Read the model definition and answer for the solid it produces. Units are mm, in the model's axes. A direction names the side the tool comes from. Give positions to 0.01 mm unless a question says otherwise; leave off trailing zeros. Loops run counter-clockwise (first coordinate to the right, second up) from the corner with the lowest first, then second, coordinate; pieces in that order, holes last. Notation, with made-up numbers: M 61.25,61.5 L 116.25,61.5 A26 cw 116.25,93.5 Z; hole C 44,-1.75 d7. An arc over 180 degrees is marked long. Return JSON: item names as keys, results as strings. Group by question number.
```python
from build123d import *

# Parameters (mm, degrees)
EXTRUDE_1_DEPTH        = 40
SKETCH_2_W             = 70
SKETCH_2_H             = 41
EXTRUDE_2_DEPTH        = 1
SKETCH_3_W             = 70
SKETCH_3_H             = 41
EXTRUDE_3_DEPTH        = 1
SKETCH_4_R             = 2.1
CUT_EXTRUDE_1_DEPTH    = 1
CUT_EXTRUDE_2_DEPTH    = 1
CUT_EXTRUDE_3_DEPTH    = 81
PATTERN_LINEAR_1_COUNT = 3
PATTERN_LINEAR_1_PITCH = 15
CUT_EXTRUDE_4_DEPTH    = 1
PATTERN_LINEAR_2_COUNT = 3
PATTERN_LINEAR_2_PITCH = 15
SKETCH_8_W             = 68
SKETCH_8_H             = 18
CUT_EXTRUDE_5_DEPTH    = 10
FILLET_1_R             = 10


with BuildPart() as part:
    # 草图1 → 凸台-拉伸1 (new body)
    with BuildSketch(Plane(origin=(0, 0, 0), x_dir=(0, 0, -1), z_dir=(1, 0, 0))):
        Polygon((0, 0), (10, 0), (10, 40), (80, 40), (80, 0), (90, 0), (90, -1), (79, -1), (79, 39), (11, 39), (11, -1), (0, -1), align=None)
    extrude(amount=EXTRUDE_1_DEPTH)

    # 草图2 → 凸台-拉伸2 (add)
    with BuildSketch(Plane(origin=(40, 0, 0), x_dir=(0, 0, -1), z_dir=(1, 0, 0))):
        with Locations((45, 19.5)):
            Rectangle(SKETCH_2_W, SKETCH_2_H)
    extrude(amount=-EXTRUDE_2_DEPTH)

    # 草图3 → 凸台-拉伸3 (add)
    with BuildSketch(Plane.ZY):
        with Locations((-45, 19.5)):
            Rectangle(SKETCH_3_W, SKETCH_3_H)
    extrude(amount=-EXTRUDE_3_DEPTH)

    # 草图4 → 切除-拉伸1 (cut)
    with BuildSketch(Plane(origin=(0, 0, 0), x_dir=(1, 0, 0), z_dir=(0, 1, 0))):
        with Locations((5, 85)):
            Circle(SKETCH_4_R)
        with Locations((35, 85)):
            Circle(SKETCH_4_R)
        with Locations((35, 5)):
            Circle(SKETCH_4_R)
        with Locations((5, 5)):
            Circle(SKETCH_4_R)
    extrude(amount=-CUT_EXTRUDE_1_DEPTH, mode=Mode.SUBTRACT)

    # 草图5 → 切除-拉伸2 (cut)
    with BuildSketch(Plane.ZY):
        with BuildLine():
            Line((-30, 15), (-30, -16.50263466))
            ThreePointArc((-30, -16.50263466), (-45, -31.50263466), (-60, -16.50263466))
            Line((-60, -16.50263466), (-60, 15))
            ThreePointArc((-60, 15), (-45, 30), (-30, 15))
        make_face()
    extrude(amount=-CUT_EXTRUDE_2_DEPTH, mode=Mode.SUBTRACT)

    # 草图6 → 切除-拉伸3 (cut, through all)
    with BuildSketch(Plane.XY.offset(-10)):
        with BuildLine():
            Line((6.5, 34), (6.5, 24))
            ThreePointArc((6.5, 24), (5, 22.5), (3.5, 24))
            Line((3.5, 24), (3.5, 34))
            ThreePointArc((3.5, 34), (5, 35.5), (6.5, 34))
        make_face()
        with BuildLine():
            Line((6.5, 16), (6.5, 6))
            ThreePointArc((6.5, 6), (5, 4.5), (3.5, 6))
            Line((3.5, 6), (3.5, 16))
            ThreePointArc((3.5, 16), (5, 17.5), (6.5, 16))
        make_face()
    cut_extrude_3 = extrude(amount=-CUT_EXTRUDE_3_DEPTH, mode=Mode.SUBTRACT)

    # 阵列(线性)1: 切除-拉伸3 ×3
    with Locations(*[(i * PATTERN_LINEAR_1_PITCH, 0, 0) for i in range(1, PATTERN_LINEAR_1_COUNT)]):
        add(cut_extrude_3, mode=Mode.SUBTRACT)

    # 草图7 → 切除-拉伸4 (cut)
    with BuildSketch(Plane(origin=(0, 40, 0), x_dir=(1, 0, 0), z_dir=(0, 1, 0))):
        with BuildLine():
            Line((7, 74), (7, 49))
            ThreePointArc((7, 49), (5.5, 47.5), (4, 49))
            Line((4, 49), (4, 74))
            ThreePointArc((4, 74), (5.5, 75.5), (7, 74))
        make_face()
        with BuildLine():
            Line((7, 41), (7, 16))
            ThreePointArc((7, 16), (5.5, 14.5), (4, 16))
            Line((4, 16), (4, 41))
            ThreePointArc((4, 41), (5.5, 42.5), (7, 41))
        make_face()
    cut_extrude_4 = extrude(amount=-CUT_EXTRUDE_4_DEPTH, mode=Mode.SUBTRACT)

    # 阵列(线性)2: 切除-拉伸4 ×3
    with Locations(*[(i * PATTERN_LINEAR_2_PITCH, 0, 0) for i in range(1, PATTERN_LINEAR_2_COUNT)]):
        add(cut_extrude_4, mode=Mode.SUBTRACT)

    # 草图8 → 切除-拉伸5 (cut)
    with BuildSketch(Plane.ZY):
        with Locations((-45, 8)):
            Rectangle(SKETCH_8_W, SKETCH_8_H)
    extrude(amount=-CUT_EXTRUDE_5_DEPTH, mode=Mode.SUBTRACT)

    # 圆角1
    fillet_1_edges = [part.edges().sort_by_distance(p)[0] for p in [
        (0.5, 17, -30.133931253),
        (0.5, 17, -59.866068747),
    ]]
    fillet(fillet_1_edges, radius=FILLET_1_R)


solid = part.part
```
1. The mould has two halves that part along X. Classify faces 1 (the cylindrical face through (3.334, -0.493, -83.722)), 2 (the flat face through (0, 32, -45)), 3 (the cylindrical face through (32.9, -0.49, -5.09)), 4 (the flat face through (20, 20, -80)): +X half, -X half, draft (parallel to the pull), parting line (faces both ways), or undercut.
2. Find section B-B (z = -5). Write down the section's boundary in (x, y).
3. Flat-ended cylindrical pins translate along their axes: P1, Ø5, axis at y = 10.5, z = -28, coming from the -X side; P2, Ø6, axis at x = 21, y = 5, coming from the +Z side; P3, Ø5, axis at y = 30, z = -48.5, coming from the -X side; P4, Ø1.5, axis at x = 35, z = -13.5, coming from the -Y side. Find the tip coordinate at first contact, or state that the pin passes through.
4. Straight lines are drawn through the part: line 1 along Z through (x, y) = (5, -0.5); line 2 along X through (y, z) = (-0.15, -5); line 3 along X through (y, z) = (27, -34). For each, find the intervals that lie inside material, in ascending order.
5. Find section A-A (z = -19.5). Write down the section's boundary in (x, y).
6. Find section C-C (x = 13). Write down the section's boundary in (y, z), and give its area (3 significant figures).
7. For faces 5 (the flat face through (20, 20, -10)), 6 (the cylindrical face through (0.493, 18.436, -61.768)), 7 (the flat face through (20, 0, -85)), 8 (the flat face through (39.2, -1, -45.2)), 9 (the flat face through (19, 19, -11)), determine the directions among +Z, -Z, +X, -X, +Y, -Y from which every point of the face is accessible in a straight line to the end or side of a thin tool.
8. Find section D-D (y = 26). State how many separate pieces and enclosed holes the cut face has, and give its area (3 significant figures).
Result:
{
 "1": {"face 1": "undercut", "face 2": "-X half", "face 3": "undercut", "face 4": "draft"},
 "2": {"outline": "M 0,-1 L 2.9,-1 L 2.9,0 L 0,0 Z; M 7.1,-1 L 32.9,-1 L 32.9,0 L 7.1,0 Z; M 37.1,-1 L 40,-1 L 40,0 L 37.1,0 Z"},
 "3": {"P1": "stops at x = 39", "P2": "stops at z = -10", "P3": "stops at x = 0", "P4": "stops at y = 39"},
 "4": {"line 1": "z = -90 to -87.1, -82.9 to -79, -11 to -7.1, -2.9 to 0", "line 2": "x = 0 to 2.9, 7.1 to 32.9, 37.1 to 40", "line 3": "x = 0 to 1, 39 to 40"},
 "5": {"outline": "M 0,17 L 1,17 L 1,39 L 4,39 L 4,40 L 0,40 Z; M 7,39 L 19,39 L 19,40 L 7,40 Z; M 22,39 L 34,39 L 34,40 L 22,40 Z; M 37,39 L 39,39 L 39,-1 L 40,-1 L 40,40 L 37,40 Z"},
 "6": {"outline": "M -1,-90 L 0,-90 L 0,-80 L 40,-80 L 40,-10 L 0,-10 L 0,0 L -1,0 L -1,-11 L 39,-11 L 39,-79 L -1,-79 Z", "area": "170 mm2"},
 "7": {"face 5": "+Z, +X, -X, +Y", "face 6": "-X, -Y", "face 7": "-Z, +X, -X, +Y", "face 8": "+Z, -Z, +X, -X, -Y", "face 9": "-Y"},
 "8": {"separate pieces": "7", "enclosed holes": "0", "area": "178 mm2"}
}
